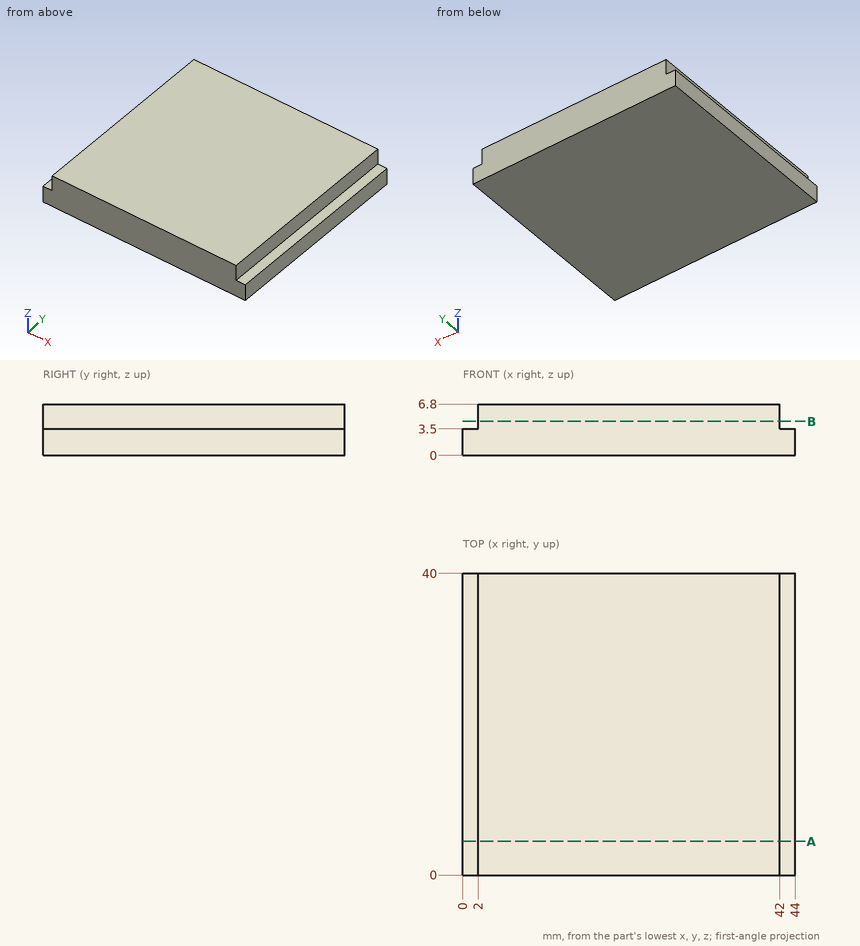
Input: dimensioned drawing with shaded views. Units: mm. Origin: part minimum x, y, z. Round coordinates to 2 decimals unless told otherwise and drop trailing zeros. Order: outer loops, then holes, each group sorted by start corner. A loop starts at its lowest first (then second) coordinate and runs counter-clockwise, first axis right, second up. Notation, with made-up numbers: (19, -32) -> (67, -32) arc R10 ccw to (67, -14) -> close; hole circle Ø10 at (84, -33.5). An arc over 180 degrees is marked (long way). One line per item, written item: value. Start each with the question number.
Q1. Pin query (flat end, axial travel): pin 1 (1 mm diameter, centred on y = 19, z = 5, fed in from +X); pin 2 (1 mm diameter, centred on y = 20.5, z = 5.5, fed in from -X); pin 3 (0.6 mm diameter, centred on x = 43, y = 21, fed in from +Z). Return the tip coordinate at first contact, or that it passes through.
Q2. Section query A-A (y = 4.5). Return the cut outline in (x, z).
Q3. Material intervals for probe 1 along X at (y, z) = (18, 6.5), sorted ascending.
Q4. Section query B-B (z = 4.5). Return the cut outline in (x, y).
Findings below:
1. pin 1: x = 42
1. pin 2: x = 2
1. pin 3: z = 3.5
2. outline: (0, 0) -> (44, 0) -> (44, 3.5) -> (42, 3.5) -> (42, 6.8) -> (2, 6.8) -> (2, 3.5) -> (0, 3.5) -> close
3. probe 1: 2 to 42
4. outline: (2, 0) -> (42, 0) -> (42, 40) -> (2, 40) -> close
